Could you check a few things on this model? Use its own coordinates, in mm. Face numbers are marked on the shaded views. A direction names the side the tool comes from. Round coordinates to 2 decimals unless told otherwise and drop trailing zeros. Write each loop counter-clockwise with the first axis right and the second up, starting at its lowest first coordinate (ties: lowest second). Pieces come first, ordered by that corner, then holes. Notation, with made-up numbers: M 83,-19.5 L 132,-19.5 A34 ccw 132,11.5 Z; hole C 9,70.25 d8. An arc over 180 degrees is marked long. One line per item, written item: value. Start each with the question number.
(1) I'm going to push flat-ended pins straight in: pin 1 Ø1 at (x, z) = (-11, 5) entering from +Y; pin 2 Ø8 at (x, z) = (-18, 13) entering from -Y; pin 3 Ø10 at (y, z) = (-21.5, 6.5) entering from -X. Where does each tip first touch, or does it pass through?
(2) I want a section at C-C on y = -18.5. Please give me the cut outline in (x, z).
(3) Which directions (+Z, -Z, +X, -X, +Y, -Y) give clear straight access to the entire face, cutting with the end or side of a thin tool? Please do the marked faces 1, 2, 3 and 4.
(4) I want a section at D-D on z = 20. Please give me the cut outline in (x, y).
(5) If I drill on L1, parallel to Y at x = -29, z = 1.5; L2, parallel to Y at x = 7.5, z = 4; L3, parallel to X at y = 36.5, z = 23.25, over which ranges is the centre line in solid material (lowest first)?
(6) I want a section at B-B on x = -18. Please give me the cut outline in (y, z), and give its area (3 significant figures).
(7) I want a section at A-A on z = 13.25. Please give me the cut outline in (x, y).
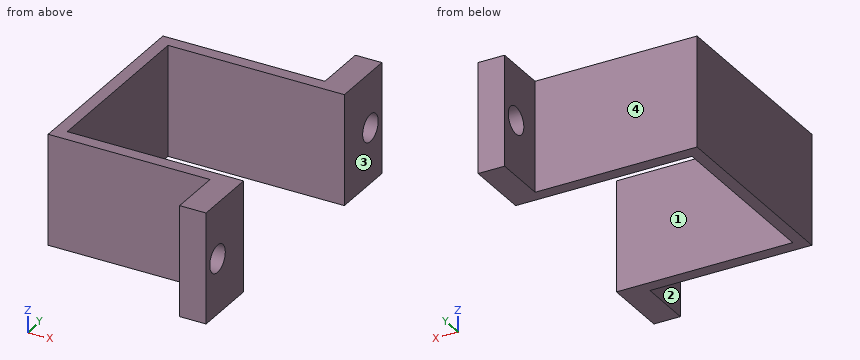
```python
from build123d import *

# Parameters (mm, degrees)
F0_W     = 6.35
F0_H     = 12.8
F1_DEPTH = 26.5
F3_D     = 6.528
F4_W     = 42.3
F4_H     = 42.3
F5_DEPTH = 26.5


with BuildPart() as f1:
    # F0 (on Top) → F1 (new body)
    with BuildSketch(Plane.XY):
        Polygon((5.245822, 36.050879), (-33.604178, 36.050879), (-33.604178, -12.149121), (5.245822, -12.149121), (11.595822, -12.149121), (11.595822, 36.050879), align=None)
        with Locations((8.420822, 42.450879)):
            Rectangle(F0_W, F0_H)
        with Locations((8.420822, -18.549121)):
            Rectangle(F0_W, F0_H)
    extrude(amount=F1_DEPTH)

    # F3 (through all)
    with Locations(Plane(origin=(5.245822, 0, 0), x_dir=(0, -1, 0), z_dir=(-1, 0, 0))):
        with Locations((-44.050879, 13.25), (20.149121, 13.25)):
            Hole(F3_D / 2)

    # F4 (on face) → F5 (cut, through all)
    with BuildSketch(Plane.XY.offset(26.5)):
        with Locations((-9.554178, 11.950879)):
            Rectangle(F4_W, F4_H)
    extrude(amount=-F5_DEPTH, mode=Mode.SUBTRACT)


solid = f1.part
```
Found:
1. pin 1: stops at y = 36.05
1. pin 2: stops at y = -12.15
1. pin 3: stops at x = 5.25
2. outline: M 5.25,0 L 11.6,0 L 11.6,10.43 L 5.25,10.43 Z; M 5.25,16.07 L 11.6,16.07 L 11.6,26.5 L 5.25,26.5 Z
3. face 1: +Z, -Z, +X
3. face 2: +Z, -Z, -X, -Y
3. face 3: +Z, -Z, +X, +Y, -Y
3. face 4: +Z, -Z, -X, +Y
4. outline: M -33.6,-12.15 L 5.25,-12.15 L 5.25,-24.95 L 11.6,-24.95 L 11.6,-9.2 L -30.7,-9.2 L -30.7,33.1 L 11.6,33.1 L 11.6,48.85 L 5.25,48.85 L 5.25,36.05 L -33.6,36.05 Z
5. L1: y = -12.15 to -9.2, 33.1 to 36.05
5. L2: y = -24.95 to -9.2, 33.1 to 48.85
5. L3: x = 5.25 to 11.6
6. outline: M -12.15,0 L -9.2,0 L -9.2,26.5 L -12.15,26.5 Z; M 33.1,0 L 36.05,0 L 36.05,26.5 L 33.1,26.5 Z
6. area: 156 mm²
7. outline: M -33.6,-12.15 L 5.25,-12.15 L 5.25,-16.89 L 11.6,-16.89 L 11.6,-9.2 L -30.7,-9.2 L -30.7,33.1 L 11.6,33.1 L 11.6,40.79 L 5.25,40.79 L 5.25,36.05 L -33.6,36.05 Z; M 5.25,-24.95 L 11.6,-24.95 L 11.6,-23.41 L 5.25,-23.41 Z; M 5.25,47.31 L 11.6,47.31 L 11.6,48.85 L 5.25,48.85 Z
